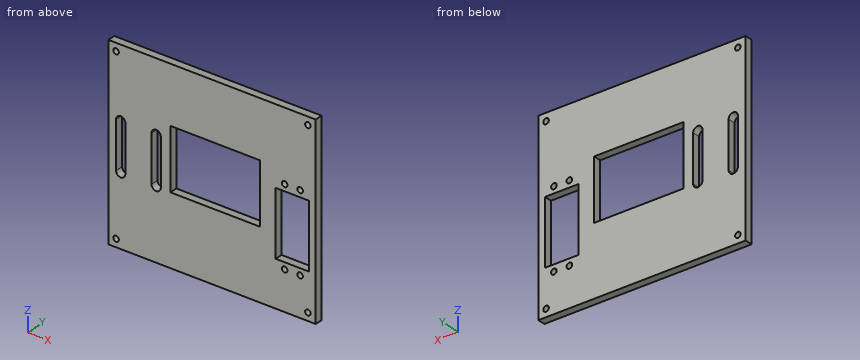
Autodesk Inventor part; units mm, degrees
ref_plane "YZ Plane" through (0, 0, 0) normal (1, 0, 0) x (0, 1, 0)
ref_plane "XZ Plane" through (0, 0, 0) normal (0, 1, 0) x (-1, 0, 0)
ref_plane "XY Plane" through (0, 0, 0) normal (0, 0, 1) x (1, 0, 0)
sketch "Sketch20" plane through (0, 0, 0) normal (0, 1, 0) x (-1, 0, 0)
  line L0 (0, 0) -> (181, 0)
  line L1 (181, 0) -> (181, 120)
  line L2 (181, 120) -> (0, 120)
  line L3 (0, 120) -> (0, 0)
  point P0 (90.5, 120)
  dimension "d122" = 181
  dimension "d123" = 120
extrude "Extrusion15" add sketch "Sketch20" along normal blind 5
sketch "Sketch22" plane through (0, 0, 0) normal (0, -1, 0) x (1, 0, 0)
  line L0 (-25.1, 70.1) -> (-5, 70.1)
  line L1 (-5, 70.1) -> (-5, 30)
  line L2 (-5, 30) -> (-25.1, 30)
  line L3 (-25.1, 30) -> (-25.1, 70.1)
  circle A0 centre (-15.05, 60) radius 1 construction
  line L4 (0, 120) -> (0, 0) construction
  circle A1 centre (-20.05, 25) radius 1.8
  circle A2 centre (-10.05, 25) radius 1.8
  circle A3 centre (-20.05, 75.1) radius 1.8
  circle A4 centre (-10.05, 75.1) radius 1.8
  line L5 (-15.05, 60) -> (0, 60) construction
  dimension "d126" = 40.1
  dimension "d127" = 20.1
  dimension "d128" = 2
  dimension "d129" = 30
  dimension "d130" = 10.05
  dimension "d134" = 5
  dimension "d135" = 5
  dimension "d136" = -5
  dimension "d137" = 5
  dimension "d138" = 5.05
  dimension "d139" = 5.05
  dimension "d140" = 5.05
  dimension "d141" = 5.05
  dimension "d142" = 3.6
  dimension "d159" = 15.05
extrude "Extrusion16" cut sketch "Sketch22" against normal blind 5
sketch "Sketch25" plane through (0, 0, 0) normal (0, -1, 0) x (1, 0, 0)
  line L0 (-181, 0) -> (-181, 120)
  line L1 (0, 0) -> (-181, 0)
  line L2 (-181, 120) -> (-134, 120)
  line L3 (-134, 120) -> (-134, 0)
  line L4 (-134, 0) -> (-181, 0)
  line L5 (-181, 0) -> (-181, 120)
  dimension "d150" = 47
extrude "Extrusion18" cut sketch "Sketch25" against normal blind 5
sketch "Sketch24" plane through (0, 0, 0) normal (0, -1, 0) x (1, 0, 0)
  circle A0 centre (-5, 5) radius 1.8
  circle A1 centre (-5, 115) radius 1.8
  circle A2 centre (-129, 115) radius 1.8
  circle A3 centre (-129, 5) radius 1.8
  line L0 (0, 0) -> (-181, 0)
  line L1 (0, 120) -> (0, 0)
  line L2 (-181, 120) -> (0, 120)
  circle A4 centre (-20.05, 25) radius 1.8
  circle A5 centre (-10.05, 25) radius 1.8
  circle A6 centre (-10.05, 75.1) radius 1.8
  line L3 (-5, 70.1) -> (-5, 30)
  line L4 (-5, 30) -> (-25.1, 30)
  line L5 (-25.1, 30) -> (-25.1, 70.1)
  line L6 (-25.1, 70.1) -> (-5, 70.1)
  circle A7 centre (-20.05, 75.1) radius 1.8
  line L7 (0, 0) -> (-134, 0)
  line L8 (0, 120) -> (0, 0)
  line L9 (-134, 120) -> (0, 120)
  line L10 (-134, 120) -> (-134, 0)
  dimension "d143" = 5
  dimension "d144" = 5
  dimension "d145" = 3.6
  dimension "d146" = 5
  dimension "d147" = 5
  dimension "d154" = 5
  dimension "d156" = 5
  dimension "d157" = 5
  dimension "d158" = 5
extrude "Extrusion17" cut sketch "Sketch24" against normal blind 5 contours A0 | A1 | A2 | A3
sketch "Sketch26" plane through (0, 0, 0) normal (0, -1, 0) x (1, 0, 0)
  circle A0 centre (-5, 5) radius 1.8
  circle A1 centre (-129, 5) radius 1.8
  circle A2 centre (-5, 115) radius 1.8
  circle A3 centre (-129, 115) radius 1.8
  line L0 (-134, 120) -> (-134, 0)
  line L1 (0, 0) -> (-134, 0)
  line L2 (0, 120) -> (0, 0)
  line L3 (-134, 120) -> (0, 120)
  circle A4 centre (-20.05, 25) radius 1.8
  circle A5 centre (-10.05, 25) radius 1.8
  circle A6 centre (-10.05, 75.1) radius 1.8
  line L4 (-5, 70.1) -> (-5, 30)
  line L5 (-5, 30) -> (-25.1, 30)
  line L6 (-25.1, 30) -> (-25.1, 70.1)
  line L7 (-25.1, 70.1) -> (-5, 70.1)
  circle A7 centre (-20.05, 75.1) radius 1.8
  line L8 (-4.5, 70.6) -> (-4.5, 29.5)
  line L9 (-4.5, 29.5) -> (-25.6, 29.5)
  line L10 (-25.6, 29.5) -> (-25.6, 70.6)
  line L11 (-25.6, 70.6) -> (-4.5, 70.6)
  dimension "d176" = 0.5
extrude "Extrusion19" cut sketch "Sketch26" against normal blind 25.4 contours L4 L5 L6 L7 | L8 L9 L10 L11
sketch "Sketch28" plane through (0, 5, 0) normal (0, 1, 0) x (1, 0, 0)
  line L0 (-49, -83.3) -> (-81, -83.3)
  arc A0 (-85, -79.3) -> (-81, -83.3) centre (-81, -79.3) ccw
  line L1 (-85, -79.3) -> (-85, -47.3)
  arc A1 (-81, -43.3) -> (-85, -47.3) centre (-81, -47.3) ccw
  line L2 (-81, -43.3) -> (-49, -43.3)
  arc A2 (-45, -47.3) -> (-49, -43.3) centre (-49, -47.3) ccw
  line L3 (-45, -47.3) -> (-45, -79.3)
  arc A3 (-49, -83.3) -> (-45, -79.3) centre (-49, -79.3) ccw
  line L4 (-81, -88.38) -> (-49, -88.38)
  arc A4 (-49, -88.38) -> (-39.92, -79.3) centre (-49, -79.3) ccw
  line L5 (-39.92, -79.3) -> (-39.92, -47.3)
  arc A5 (-39.92, -47.3) -> (-49, -38.22) centre (-49, -47.3) ccw
  line L6 (-49, -38.22) -> (-81, -38.22)
  arc A6 (-81, -38.22) -> (-90.08, -47.3) centre (-81, -47.3) ccw
  line L7 (-90.08, -47.3) -> (-90.08, -79.3)
  arc A7 (-90.08, -79.3) -> (-81, -88.38) centre (-81, -79.3) ccw
  point P0 (0, 0)
  dimension "d165" = 5.08
extrude "Extrusion21" cut sketch "Sketch28" against normal blind 25.4 contours L0 A0 L1 A1 L2 A2 L3 A3 | A7 L7 A6 L6 A5 L5 A4 L4
sketch "Sketch29" plane through (0, 5, 0) normal (0, 1, 0) x (1, 0, 0)
  arc A0 (-106.08, -75) -> (-100.08, -75) centre (-103.08, -75) ccw
  line L0 (-100.08, -45) -> (-100.08, -75)
  line L1 (-106.08, -75) -> (-106.08, -45)
  arc A1 (-129, -75) -> (-123, -75) centre (-126, -75) ccw
  line L2 (-123, -45) -> (-123, -75)
  line L3 (-129, -75) -> (-129, -45)
  arc A2 (-123, -45) -> (-129, -45) centre (-126, -45) ccw
  arc A3 (-100.08, -45) -> (-106.08, -45) centre (-103.08, -45) ccw
  line L4 (-39.92, -47.3) -> (-39.92, -79.3)
  arc A4 (-49, -88.38) -> (-39.92, -79.3) centre (-49, -79.3) ccw
  line L5 (-49, -88.38) -> (-81, -88.38)
  arc A5 (-90.08, -79.3) -> (-81, -88.38) centre (-81, -79.3) ccw
  line L6 (-90.08, -79.3) -> (-90.08, -47.3)
  arc A6 (-81, -38.22) -> (-90.08, -47.3) centre (-81, -47.3) ccw
  line L7 (-81, -38.22) -> (-49, -38.22)
  arc A7 (-39.92, -47.3) -> (-49, -38.22) centre (-49, -47.3) ccw
  line L8 (-25.6, -29.5) -> (-4.5, -29.5)
  line L9 (-4.5, -29.5) -> (-4.5, -70.6)
  line L10 (-4.5, -70.6) -> (-25.6, -70.6)
  line L11 (-25.6, -70.6) -> (-25.6, -29.5)
  circle A8 centre (-5, -5) radius 1.8
  circle A9 centre (-129, -5) radius 1.8
  circle A10 centre (-5, -115) radius 1.8
  circle A11 centre (-129, -115) radius 1.8
  line L12 (-134, 0) -> (-134, -120)
  line L13 (-134, -120) -> (0, -120)
  line L14 (0, -120) -> (0, 0)
  line L15 (0, 0) -> (-134, 0)
  circle A12 centre (-20.05, -75.1) radius 1.8
  circle A13 centre (-10.05, -75.1) radius 1.8
  circle A14 centre (-10.05, -25) radius 1.8
  circle A15 centre (-20.05, -25) radius 1.8
  line L16 (-129, -60) -> (-134, -60) construction
  line L17 (-106.08, -60) -> (-123, -60) construction
  line L18 (-129, -45) -> (-126, -45) construction
  line L19 (-103.08, -45) -> (-106.08, -45) construction
  dimension "d139" = 5.05
  dimension "d168" = 30
  dimension "d169" = 5
  dimension "d170" = 10
  dimension "d171" = 6
  dimension "d172" = 6
  dimension "d173" = 3
extrude "Extrusion22" cut sketch "Sketch29" against normal blind 25.4 contours L1 A3 L0 A0 | L3 A2 L2 A1
sketch "Sketch30" plane through (0, 5, 0) normal (0, 1, 0) x (1, 0, 0)
  arc A0 (-100.08, -45) -> (-106.08, -45) centre (-103.08, -45) ccw
  line L0 (-100.08, -45) -> (-100.08, -75)
  arc A1 (-106.08, -75) -> (-100.08, -75) centre (-103.08, -75) ccw
  line L1 (-106.08, -75) -> (-106.08, -45)
  arc A2 (-123, -45) -> (-129, -45) centre (-126, -45) ccw
  line L2 (-123, -45) -> (-123, -75)
  arc A3 (-129, -75) -> (-123, -75) centre (-126, -75) ccw
  line L3 (-129, -75) -> (-129, -45)
  line L4 (-39.92, -47.3) -> (-39.92, -79.3)
  arc A4 (-49, -88.38) -> (-39.92, -79.3) centre (-49, -79.3) ccw
  line L5 (-49, -88.38) -> (-81, -88.38)
  arc A5 (-90.08, -79.3) -> (-81, -88.38) centre (-81, -79.3) ccw
  line L6 (-90.08, -79.3) -> (-90.08, -47.3)
  arc A6 (-81, -38.22) -> (-90.08, -47.3) centre (-81, -47.3) ccw
  line L7 (-81, -38.22) -> (-49, -38.22)
  arc A7 (-39.92, -47.3) -> (-49, -38.22) centre (-49, -47.3) ccw
  line L8 (-25.6, -29.5) -> (-4.5, -29.5)
  line L9 (-4.5, -29.5) -> (-4.5, -70.6)
  line L10 (-4.5, -70.6) -> (-25.6, -70.6)
  line L11 (-25.6, -70.6) -> (-25.6, -29.5)
  circle A8 centre (-5, -5) radius 1.8
  circle A9 centre (-129, -5) radius 1.8
  circle A10 centre (-5, -115) radius 1.8
  circle A11 centre (-129, -115) radius 1.8
  line L12 (-134, 0) -> (-134, -120)
  line L13 (-134, -120) -> (0, -120)
  line L14 (0, -120) -> (0, 0)
  line L15 (0, 0) -> (-134, 0)
  circle A12 centre (-20.05, -75.1) radius 1.8
  circle A13 centre (-10.05, -75.1) radius 1.8
  circle A14 centre (-10.05, -25) radius 1.8
  circle A15 centre (-20.05, -25) radius 1.8
extrude "Extrusion23" add sketch "Sketch30" against normal blind 5 contours L4 A4 L5 A5 L6 A6 L7 A7
sketch "Sketch31" plane through (0, 5, 0) normal (0, 1, 0) x (1, 0, 0)
  arc A0 (-100.08, -45) -> (-106.08, -45) centre (-103.08, -45) ccw
  line L0 (-100.08, -45) -> (-100.08, -75)
  arc A1 (-106.08, -75) -> (-100.08, -75) centre (-103.08, -75) ccw
  line L1 (-106.08, -75) -> (-106.08, -45)
  arc A2 (-123, -45) -> (-129, -45) centre (-126, -45) ccw
  line L2 (-123, -45) -> (-123, -75)
  arc A3 (-129, -75) -> (-123, -75) centre (-126, -75) ccw
  line L3 (-129, -75) -> (-129, -45)
  line L4 (-25.6, -29.5) -> (-4.5, -29.5)
  line L5 (-4.5, -29.5) -> (-4.5, -70.6)
  line L6 (-4.5, -70.6) -> (-25.6, -70.6)
  line L7 (-25.6, -70.6) -> (-25.6, -29.5)
  circle A4 centre (-5, -5) radius 1.8
  circle A5 centre (-129, -5) radius 1.8
  circle A6 centre (-5, -115) radius 1.8
  circle A7 centre (-129, -115) radius 1.8
  line L8 (-134, 0) -> (-134, -120)
  line L9 (-134, -120) -> (0, -120)
  line L10 (0, -120) -> (0, 0)
  line L11 (0, 0) -> (-134, 0)
  circle A8 centre (-20.05, -75.1) radius 1.8
  circle A9 centre (-10.05, -75.1) radius 1.8
  circle A10 centre (-10.05, -25) radius 1.8
  circle A11 centre (-20.05, -25) radius 1.8
  line L12 (-4.246, -29.246) -> (-25.854, -29.246)
  line L13 (-25.854, -29.246) -> (-25.854, -70.854)
  line L14 (-25.854, -70.854) -> (-4.246, -70.854)
  line L15 (-4.246, -70.854) -> (-4.246, -29.246)
  dimension "d179" = 0.254
extrude "Extrusion24" cut sketch "Sketch31" against normal blind 5 contours L4 L5 L6 L7 | L15 L14 L13 L12
sketch "Sketch32" plane through (0, 5, 0) normal (0, 1, 0) x (1, 0, 0)
  line L0 (-93.9, -44.81) -> (-93.9, -83.21)
  line L1 (-93.9, -83.51) -> (-36.1, -83.51)
  line L2 (-93.9, -83.51) -> (-36.1, -83.51)
  line L3 (-36.1, -83.21) -> (-36.1, -44.81)
  line L4 (-93.9, -83.21) -> (-36.1, -83.21)
  line L5 (-36.1, -44.81) -> (-93.9, -44.81)
  line L6 (-36.1, -44.51) -> (-93.9, -44.51)
  line L7 (-36.1, -44.51) -> (-93.9, -44.51)
  line L8 (-36.1, -83.51) -> (-93.9, -83.51)
  line L9 (-93.9, -83.51) -> (-93.9, -44.51)
  line L10 (-93.9, -44.51) -> (-36.1, -44.51)
  line L11 (-36.1, -44.51) -> (-36.1, -83.51)
  point P0 (0, 0)
extrude "Extrusion25" cut sketch "Sketch32" against normal blind 5
properties part number "tamiya_chassis_3DPrint"
For this review, take the finished solid that the model builds, in its own axes (mm). Round coordinates to 2 decimals unless told otherwise and drop trailing zeros. Write each loop counter-clockwise with the first axis right and the second up, starting at its lowest first coordinate (ties: lowest second). Pieces come first, ordered by that corner, then holes. Notation, with made-up numbers: (88.5, 35.25) -> (128.5, 35.25) arc R31 ccw to (128.5, 61.25) -> close; hole circle Ø9 at (36, 34). An arc over 180 degrees is marked (long way). Use CSV: the item, a comma, the result in double quotes.
(1) Clearance check with flat-ended pins moving along their axes: P1, Ø3, axis at x = -10.05, z = 25, coming from the -Y side; P2, Ø4, axis at x = -20.05, z = 75.1, coming from the -Y side. State where each tip first meets the part, or that it passes through.
Computed values:
P1,"through"
P2,"y = 0"
(2) To check wall thickness, follow L1, parallel to Z at x = -5, y = 1.35; L2, parallel to X at y = 1.45, z = 115; L3, parallel to X at y = 0.4, z = 70.5. State the ranges of each line that lie inside material, in increasing order. Write a range as [from, to].
Computed values:
L1,"[0, 3.2], [6.8, 29.25], [70.85, 113.2], [116.8, 120]"
L2,"[-134, -130.8], [-127.2, -6.8], [-3.2, 0]"
L3,"[-134, -129], [-123, -106.08], [-100.08, -93.9], [-36.1, -25.85], [-4.25, 0]"
(3) Consider section B-B, the plane z = 53.5. Give the boundary of the cut face in (x, y), plus the area to 3 significant figures.
Computed values:
outline,"(-134, 0) -> (-129, 0) -> (-129, 5) -> (-134, 5) -> close; (-123, 0) -> (-106.08, 0) -> (-106.08, 5) -> (-123, 5) -> close; (-100.08, 0) -> (-93.9, 0) -> (-93.9, 5) -> (-100.08, 5) -> close; (-36.1, 0) -> (-25.85, 0) -> (-25.85, 5) -> (-36.1, 5) -> close; (-4.25, 0) -> (0, 0) -> (0, 5) -> (-4.25, 5) -> close"
area,"213 mm²"
(4) Consider section D-D, the plane z = 25. Give the boundary of the cut face in (x, y).
Computed values:
outline,"(-134, 0) -> (-21.85, 0) -> (-21.85, 5) -> (-134, 5) -> close; (-18.25, 0) -> (-11.85, 0) -> (-11.85, 5) -> (-18.25, 5) -> close; (-8.25, 0) -> (0, 0) -> (0, 5) -> (-8.25, 5) -> close"
(5) Consider section A-A, the plane x = -10.05. Give the boundary of the cut face in (y, z), plus the area to 3 significant figures.
Computed values:
outline,"(0, 0) -> (5, 0) -> (5, 23.2) -> (0, 23.2) -> close; (0, 26.8) -> (5, 26.8) -> (5, 29.25) -> (0, 29.25) -> close; (0, 70.85) -> (5, 70.85) -> (5, 73.3) -> (0, 73.3) -> close; (0, 76.9) -> (5, 76.9) -> (5, 120) -> (0, 120) -> close"
area,"356 mm²"
(6) Consider section C-C, the plane x = -103.08. Give the boundary of the cut face in (y, z).
Computed values:
outline,"(0, 0) -> (5, 0) -> (5, 42) -> (0, 42) -> close; (0, 78) -> (5, 78) -> (5, 120) -> (0, 120) -> close"
